Here's the drawing with two shaded views (mm, measured from the low corner). I have some questions. Round coordinates to 2 decimals unless told otherwise and drop trailing zeros. Loops run counter-clockwise (first coordinate to the right, second up) from the corner with the lowest first, then second, coordinate; pieces in that order, holes last. Notation, with made-up numbers: M -27.5,65.5 L 1.5,65.5 A16 ccw 1.5,81.5 Z; hole C 5,-20 d11. An arc over 180 degrees is marked long. Write each question's results on one line, items separated by ' | '. Start each with the question number.
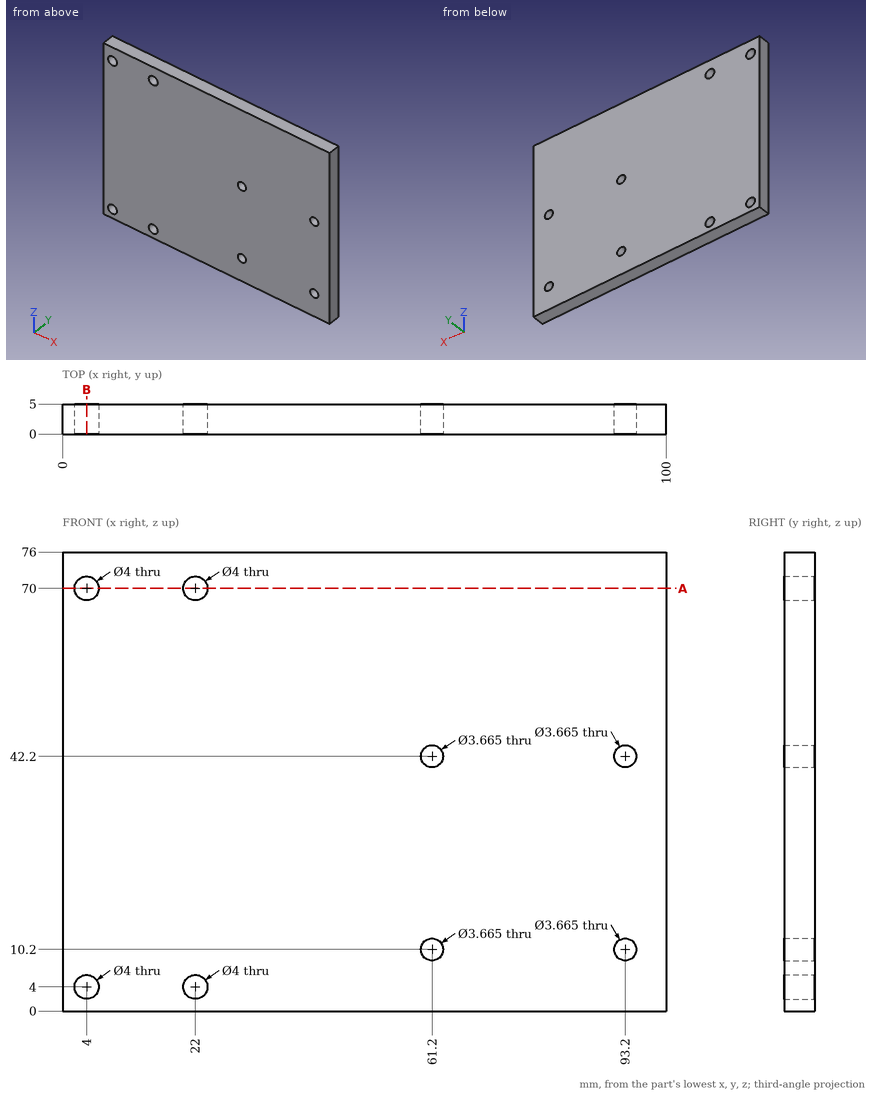
Item 1: I need wall thicknesses on L1, parallel to Z at x = 61.2, y = 2; L2, parallel to X at y = 2.95, z = 70; L3, parallel to X at y = 1.35, z = 42.2. Which ranges of each line are inside material? Lowest first, please.
Item 2: I'm going to push a flat-ended pin straight in: pin 1 (6 mm diameter, centred on x = 34.5, z = 15.5, fed in from -Y). Where does the tip first touch, or does it pass through?
Item 3: If we section it at B-B on x = 4: Please give me the cut outline in (y, z).
Item 4: If we section it at A-A on z = 70: Please give me the cut outline in (x, y).
Numbers:
1) L1: 0 to 8.37, 12.03 to 40.37, 44.03 to 76 | L2: 0 to 2, 6 to 20, 24 to 100 | L3: 0 to 59.37, 63.03 to 91.37, 95.03 to 100
2) pin 1: y = 0
3) outline: M 0,0 L 5,0 L 5,2 L 0,2 Z; M 0,6 L 5,6 L 5,68 L 0,68 Z; M 0,72 L 5,72 L 5,76 L 0,76 Z
4) outline: M 0,0 L 2,0 L 2,5 L 0,5 Z; M 6,0 L 20,0 L 20,5 L 6,5 Z; M 24,0 L 100,0 L 100,5 L 24,5 Z
